Read the model definition and answer for the solid it produces. Units are mm, in the model's axes. A direction names the side the tool comes from. Coordinates: 2 decimals unless noted, no trailing zeros. Loops run counter-clockwise (first coordinate to the right, second up) from the corner with the lowest first, then second, coordinate; pieces in that order, holes last. Notation, with made-up numbers: (60, -19) -> (74, -19) arc R11 cw to (74, -1) -> close; hole circle Ø1 at (32, -5.5). An arc over 180 degrees is marked (long way). Answer as a JSON object with one key per item and string values. Group by question number.
Q1. Straight lines are drawn through the part: line 1 along Z through (x, y) = (-1.45, 14.5); line 2 along Y through (x, z) = (-0.95, 22); line 3 along Y through (x, z) = (-0.55, 114.5). For each, find the intervals that lie inside material, in ascending order. Write a range as [from, to].
Q2. The part is cut by section B-B on x = -1.5. Write down the section's boundary in (y, z).
Q3. The part is cut by section D-D on z = 37. Write down the section's boundary in (x, y).
Q4. Each of these flat-tipped pins is pushed along its axis until it touches: P1, Ø1, axis at x = -1, z = 92.5, coming from the -Y side; P2, Ø4, axis at y = 19.5, z = 18.5, coming from the +X side; P3, Ø0.9, axis at x = -1.5, z = 1, coming from the -Y side. Where does it stop, or does it pass through?
Q5. Determine the mould class of faces 4 (the cylindrical face through (-1.479, 97.734, 37.26)), 5 (the flat face through (-2, 68, -3)), 6 (the cylindrical face through (-1.479, 4.058, 58.112)) for opening direction Z: released by +Z, released by -Z, zero draft, split by the parting line, or undercut.
Q6. For faces 1 (the flat face through (-1, 33, 117)), 2 (the flat face through (-2, 69, 121)), 3 (the flat face through (-1, 33, 1)), determine the directions among +Z, -Z, +X, -X, +Y, -Y from which every point of the face is accessible in a straight line to the end or side of a thin tool.
Q7. The part is cut by section A-A on z = 22. Write down the section's boundary in (x, y).
Q8. The part is cut by section C-C on y = 20. Write down the section's boundary in (x, z), and give its area (3 significant figures).
from build123d import *

# Parameters (mm, degrees)
IMPORTED_START          = -3
IMPORTED_BODY_4_1_DEPTH = 3
SKETCH_1_R              = 2
CUT_EXTRUDE_1_DEPTH     = 3
SKETCH_2_W              = 30
SKETCH_2_H              = 3
SKETCH_2_W_2            = 3
SKETCH_2_H_2            = 30
EXTRUDE_1_DEPTH         = 3
CUT_EXTRUDE_2_DEPTH     = 3


# Read off the part's stored shape, not the designer's step: 基体零件-零件4-1
with BuildPart() as part:
    # 基体零件-零件4-1 outline → 基体零件-零件4-1 (new body)
    with BuildSketch(Plane.YZ.offset(IMPORTED_START)):
        Polygon((-3, -3), (0, -3), (0, 0), (9.999598957, 0), (9.999598957, 3), (20.000401043, 3), (20.000401043, 0), (30, 0), (30, -3), (52, -3), (52, 0), (82, 0), (82, -3), (104, -3), (104, 19), (101, 19), (101, 49), (104, 49), (104, 69), (101, 69), (101, 99), (104, 99), (104, 121), (82, 121), (82, 118), (52, 118), (52, 121), (30, 121), (30, 118), (20.000401043, 118), (20.000401043, 115), (9.999598957, 115), (9.999598957, 118), (0, 118), (0, 121), (-3, 121), (-3, 99), (0, 99), (0, 69), (-3, 69), (-3, 49), (0, 49), (0, 19), (-3, 19), align=None)
    extrude(amount=IMPORTED_BODY_4_1_DEPTH)

    # 草图1 → 切除-拉伸1 (cut)
    with BuildSketch(Plane(origin=(0, 0, 0), x_dir=(0, 0, -1), z_dir=(1, 0, 0))):
        with Locations((-96, 95.751318052)):
            Circle(SKETCH_1_R)
        with Locations((-81, 95.751318052)):
            Circle(SKETCH_1_R)
        with Locations((-37, 95.751318052)):
            Circle(SKETCH_1_R)
        with Locations((-22, 95.751318052)):
            Circle(SKETCH_1_R)
    extrude(amount=-CUT_EXTRUDE_1_DEPTH, mode=Mode.SUBTRACT)

    # 草图2 → 凸台-拉伸1 (add)
    with BuildSketch(Plane(origin=(0, 0, 0), x_dir=(0, 0, -1), z_dir=(1, 0, 0))):
        with Locations((-84, 102.5)):
            Rectangle(SKETCH_2_W, SKETCH_2_H)
        with Locations((-34, 102.5)):
            Rectangle(SKETCH_2_W, SKETCH_2_H)
        with Locations((-119.5, 67)):
            Rectangle(SKETCH_2_W_2, SKETCH_2_H_2)
        with Locations((1.5, 67)):
            Rectangle(SKETCH_2_W_2, SKETCH_2_H_2)
    extrude(amount=-EXTRUDE_1_DEPTH)

    # 草图3 → 切除-拉伸2 (cut)
    with BuildSketch(Plane(origin=(0, 0, 0), x_dir=(0, 0, -1), z_dir=(1, 0, 0))):
        with BuildLine():
            Line((-112.520298482, 33), (-121, 33))
            Line((-121, 33), (-121, -3))
            Line((-121, -3), (3, -3))
            Line((3, -3), (3, 33))
            Line((3, 33), (-5.479701518, 33))
            ThreePointArc((-5.479701518, 33), (-59, 4.051408541), (-112.520298482, 33))
        make_face()
    extrude(amount=-CUT_EXTRUDE_2_DEPTH, mode=Mode.SUBTRACT)


solid = part.part
Final values:
{
 "1": {"line 1": "z = [23.97, 94.03]", "line 2": "y = [15.84, 93.75], [97.75, 104]", "line 3": "y = [33, 104]"},
 "2": {"outline": "(33, -3) -> (104, -3) -> (104, 121) -> (33, 121) -> (33, 112.52) arc R63.95 ccw to (33, 5.48) -> close; hole circle Ø4 at (95.75, 22); hole circle Ø4 at (95.75, 37); hole circle Ø4 at (95.75, 81); hole circle Ø4 at (95.75, 96)"},
 "3": {"outline": "(-3, 7.95) -> (0, 7.95) -> (0, 93.75) -> (-3, 93.75) -> close; (-3, 97.75) -> (0, 97.75) -> (0, 104) -> (-3, 104) -> close"},
 "4": {"P1": "stops at y = 13.22", "P2": "stops at x = 0", "P3": "stops at y = 33"},
 "5": {"face 4": "undercut", "face 5": "released by -Z", "face 6": "split by the parting line"},
 "6": {"face 1": "+Z, +X, -X, -Y", "face 2": "+Z, +X, -X, +Y, -Y", "face 3": "-Z, +X, -X, -Y"},
 "7": {"outline": "(-3, 15.84) -> (0, 15.84) -> (0, 93.75) -> (-3, 93.75) -> close; (-3, 97.75) -> (0, 97.75) -> (0, 104) -> (-3, 104) -> close"},
 "8": {"outline": "(-3, 16.75) -> (0, 16.75) -> (0, 101.25) -> (-3, 101.25) -> close", "area": "254 mm2"}
}
